Model file for the job. Use its own axes, mm. A direction names the side the tool comes from. Coordinates: 2 decimals unless noted, no trailing zeros. Order: outer loops, then holes, each group sorted by start corner. A loop starts at its lowest first (then second) coordinate and runs counter-clockwise, first axis right, second up. Notation, with made-up numbers: (60.5, -1.5) - (117.5, -1.5) arc R14 cw to (117.5, 15.5) - close; hole circle Ø5 at (7.5, 0.25). An arc over 180 degrees is marked (long way). Put each result on its own line as item: value. Start each with the question number.
```python
from build123d import *

# Parameters (mm, degrees)
F0_R     = 54.4188392039
F0_R_2   = 41.2465801868
F1_DEPTH = 66.04
F2_W     = 151.658192277
F2_H     = 95.9565676749
F3_DEPTH = 25.4
F4_DEPTH = 50.8
F5_W     = 11.7014325224
F5_H     = 33.2940161884
F6_DEPTH = 101.6
F8_DEPTH = 25.4


with BuildPart() as f1:
    # F0 (on Top) → F1 (new body)
    with BuildSketch(Plane.XY):
        with Locations((75.9313777089, 0)):
            Circle(F0_R)
        with Locations((75.9313777089, 0)):
            Circle(F0_R_2, mode=Mode.SUBTRACT)
    extrude(amount=F1_DEPTH)

    # F2 (on Top) → F3 (join)
    with BuildSketch(Plane.XY):
        with Locations((-0.2903938293, -6.1472672969)):
            Rectangle(F2_W, F2_H)
    extrude(amount=F3_DEPTH)

    # F4 (cut): a face of the model
    f4_faces = [f1.faces().sort_by_distance(p)[0] for p in [
        (58.2134002608, 0, 25.4),
    ]]
    extrude(f4_faces, amount=-F4_DEPTH, mode=Mode.SUBTRACT)

    # F5 (on face) → F6 (join)
    with BuildSketch(Plane(origin=(-76.1194899678, 0, 0), x_dir=(0, -1, 0), z_dir=(-1, 0, 0))):
        with Locations((0.2965510357, 42.0470080942)):
            Rectangle(F5_W, F5_H)
    extrude(amount=-F6_DEPTH)

    # F7 (on face) → F8 (cut)
    with BuildSketch(Plane.XZ.offset(6.1472672969)):
        Polygon((-76.1194899678, 25.4), (-52.8771914542, 25.4), (21.8608574129, 58.6940161884), (-76.1194899678, 58.6940161884), align=None)
    extrude(amount=-F8_DEPTH, mode=Mode.SUBTRACT)


solid = f1.part
```
Item 1: Flat gauge pins, fed straight in: pin 1 Ø2 at (x, z) = (75, 14.5) entering from -Y; pin 2 Ø5 at (y, z) = (28.5, 18) entering from +X; pin 3 Ø1.5 at (y, z) = (28, 26) entering from -X; pin 4 Ø3 at (x, z) = (34, 23.5) entering from -Y. Where does each tip first touch, or does it go through?
Item 2: Pull direction X, two halves, no side cores. Call faces 4 (the face through (127.837, 16.346, 39.895)), 5 (the face through (34.725, 1.814, 32.558)), 6 (the face through (1, -6.147, 34)): pulls with the +X half, pulls with the -X half, needs draft (parallel to the pull), parting line crosses it, or undercut.
Item 3: Wall check: line 1 along X through (y, z) = (-14.5, 59); line 2 along Y through (x, z) = (5, 25); line 3 along Z through (x, y) = (10.5, -32). Give the ranges that are in metal, low to high.
Item 4: Slice it at B-B, the plane x = 82.5. Give the cut face in (y, z), plus the area to 3 significant figures.
Item 5: Slice it at A-A, the plane y = 0. Give the cut face in (x, z), plus the area to 3 significant figures.
Item 6: Slice it at C-C, the plane z = 54. Give the cut face in (x, y).
Item 7: Slice it at D-D, the plane y = -35. Give the cut face in (x, z), plus the area to 3 significant figures.
Item 8: 3-axis set-ups, long thin cutter, end or side, ignore diameter. For faces 1 (the face through (-20, -16, 25.4)), 2 (the face through (-4, -54.126, 13)), 3 (the face through (-18, 41.831, 13)): which of +Z, -Z, +X, -X, +Y, -Y reach the whole face in a straight line?
Here are the results:
1. pin 1: stops at y = -54.42
1. pin 2: stops at x = 123.74
1. pin 3: stops at x = -76.12
1. pin 4: stops at y = -54.13
2. face 4: parting line crosses it
2. face 5: undercut
2. face 6: needs draft
3. line 1: x = 23.48 to 37.32, 114.55 to 128.38
3. line 2: y = -54.13 to 41.83
3. line 3: z = 0 to 25.4
4. outline: (-54.02, 0) - (-40.72, 0) - (-40.72, 66.04) - (-54.02, 66.04) - close; (40.72, 0) - (54.02, 0) - (54.02, 66.04) - (40.72, 66.04) - close
4. area: 1,760 mm^2
5. outline: (-76.12, 0) - (34.68, 0) - (34.68, 66.04) - (21.51, 66.04) - (21.51, 58.69) - (21.86, 58.69) - (-52.88, 25.4) - (-76.12, 25.4) - close; (117.18, 0) - (130.35, 0) - (130.35, 66.04) - (117.18, 66.04) - close
5. area: 5,450 mm^2
6. outline: (11.32, -6.15) - (21.86, -6.15) arc R54.42 ccw (long way) to (21.8, 5.55) - (11.32, 5.55) - close; hole circle Ø82.49 at (75.93, 0)
7. outline: (-76.12, 0) - (54.11, 0) - (54.11, 66.04) - (34.26, 66.04) - (34.26, 25.4) - (-76.12, 25.4) - close; (97.76, 0) - (117.6, 0) - (117.6, 66.04) - (97.76, 66.04) - close
7. area: 5,420 mm^2
8. face 1: +Z, -X
8. face 2: +Z, -Z, -X, -Y
8. face 3: +Z, -Z, -X, +Y
